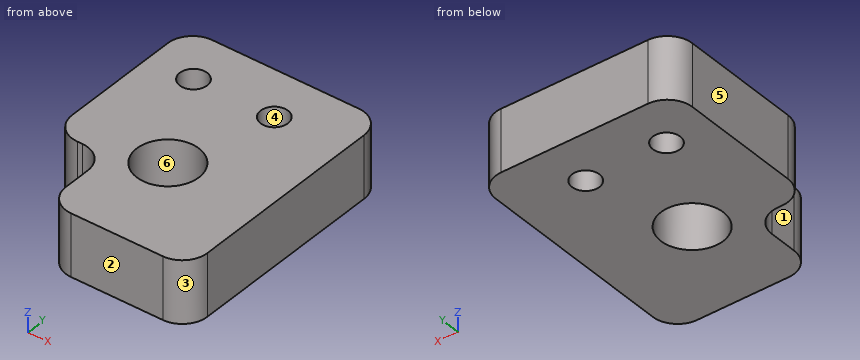
```python
from build123d import *

# Parameters (mm, degrees)
F0_R     = 2.5
F0_R_2   = 1.1
F1_DEPTH = 5
F2_R     = 2


with BuildPart() as f1:
    # F0 (on Top) → F1 (new body)
    with BuildSketch(Plane.XY):
        Polygon((7.9, 8.3929710358), (0, 8.3929710358), (-7.9, 8.3929710358), (-7.9, -5.3654396906), (-3.4737212118, -5.3654396906), (-3.4737212118, -11.6070289642), (0, -11.6070289642), (7.9, -11.6070289642), align=None)
        with Locations((0, -3.6070289642)):
            Circle(F0_R, mode=Mode.SUBTRACT)
        with Locations((-4.25, 4.3929710358)):
            Circle(F0_R_2, mode=Mode.SUBTRACT)
        with Locations((2.25, 4.3929710358)):
            Circle(F0_R_2, mode=Mode.SUBTRACT)
    extrude(amount=F1_DEPTH)

    # F2
    f2_edges = [f1.edges().sort_by_distance(p)[0] for p in [
        (7.9, -11.607029, 2.5),
        (7.9, 8.392971, 2.5),
        (-3.473721, -11.607029, 2.5),
        (-7.9, 8.392971, 2.5),
        (-7.9, -5.36544, 2.5),
        (-3.473721, -5.36544, 2.5),
    ]]
    fillet(f2_edges, radius=F2_R)


solid = f1.part
```
Verification items for the finished model (mm, model axes). Face numbers are marked on the shaded views. A direction names the side the tool comes from. Give positions to 0.01 mm unless a question says otherwise; leave off trailing zeros. Loops run counter-clockwise (first coordinate to the right, second up) from the corner with the lowest first, then second, coordinate; pieces in that order, holes last.
1. Thickness scan on line 1 (Y direction, x = 2.25, z = 2.65); line 2 (Y direction, x = 0, z = 1.7); line 3 (Y direction, x = -4.5, z = 1.5). Record the ranges inside material, lowest first.
2. Set-up check for the marked faces 1 and 2: record each of +Z, -Z, +X, -X, +Y, -Y from which the full face is reachable in a straight line by a thin tool's end or side.
3. Section check D-D, the plane z = 3.85. Enter the section's corners in (x, y), then the cut area to 3 significant figures.
4. Section check B-B, the plane y = -1.5. Enter the section's corners in (x, z), then the cut area to 3 significant figures.
5. Go/stop test with flat-tipped pins: pin 1 Ø3 at (x, y) = (2.25, 4.39) entering from -Z; pin 2 Ø1.1 at (y, z) = (-8.5, 3.5) entering from -X. Record where each tip stops, or that it passes through.
6. Section check A-A, the plane x = 0. Enter the section's corners in (y, z).
7. Section check C-C, the plane x = 2.25. Enter the section's corners in (y, z), then the cut area to 3 significant figures.
8. Mould release check, pull along Y, two halves, no side actions. Record for the marked faces 3, 4, 5 and 6: released by +Y, released by -Y, zero draft, split by the parting line, or undercut.
Geometry says:
1. line 1: y = -11.61 to -4.7, -2.52 to 3.29, 5.49 to 8.39
1. line 2: y = -11.61 to -6.11, -1.11 to 8.39
1. line 3: y = -5.62 to 3.32, 5.46 to 8.39
2. face 1: +Z, -Z, -X, -Y
2. face 2: +Z, -Z, +X, -X, -Y
3. outline: (-7.9, -3.37) arc R2 ccw to (-5.9, -5.37) - (-5.47, -5.37) arc R2 cw to (-3.47, -7.37) - (-3.47, -9.61) arc R2 ccw to (-1.47, -11.61) - (5.9, -11.61) arc R2 ccw to (7.9, -9.61) - (7.9, 6.39) arc R2 ccw to (5.9, 8.39) - (-5.9, 8.39) arc R2 ccw to (-7.9, 6.39) - close; hole circle Ø2.2 at (-4.25, 4.39); hole circle Ø5 at (0, -3.61); hole circle Ø2.2 at (2.25, 4.39)
3. area: 258 mm2
4. outline: (-7.9, 0) - (-1.35, 0) - (-1.35, 5) - (-7.9, 5) - close; (1.35, 0) - (7.9, 0) - (7.9, 5) - (1.35, 5) - close
4. area: 65.5 mm2
5. pin 1: stops at z = 0
5. pin 2: stops at x = -3.47
6. outline: (-11.61, 0) - (-6.11, 0) - (-6.11, 5) - (-11.61, 5) - close; (-1.11, 0) - (8.39, 0) - (8.39, 5) - (-1.11, 5) - close
7. outline: (-11.61, 0) - (-4.7, 0) - (-4.7, 5) - (-11.61, 5) - close; (-2.52, 0) - (3.29, 0) - (3.29, 5) - (-2.52, 5) - close; (5.49, 0) - (8.39, 0) - (8.39, 5) - (5.49, 5) - close
7. area: 78.1 mm2
8. face 3: released by -Y
8. face 4: undercut
8. face 5: zero draft
8. face 6: undercut
